Autodesk Fusion 360 part; units mm, degrees
sketch "Sketch1" plane through (0, 0, 0) normal (0, 0, 1) x (1, 0, 0) in component "Case "
  line L0 (0, 0) -> (117.5, 0)
  line L1 (117.5, 0) -> (117.5, -47.5)
  line L2 (117.5, -47.5) -> (62.4309, -113.1288)
  line L3 (0, 0) -> (0, -75)
  line L4 (0, -75) -> (62.4309, -113.1288)
  line L5 (0, -66.2119) -> (67.3065, -107.3183)
  line L6 (55.9577, -109.1753) -> (117.5, -35.8321)
  line L7 (0, -7.5) -> (117.5, -7.5)
  line L8 (110, 0) -> (110, -56.4382)
  line L9 (117.5, -47.5) -> (0, -47.5)
  dimension "d3" = 140
  dimension "d11" = 7.5
  dimension "d12" = 7.5
  dimension "d13" = 7.5
  dimension "d14" = 7.5
  dimension "d15" = 110
  dimension "d16" = 47.5
  dimension "d17" = 18.7119
  dimension "d18" = 75
extrude "Extrude1" add sketch "Sketch1" along normal blind 5
extrude "Extrude2" cut 1 faces at (39.1667, -40.8333, 5) along direction (0, 0, -1) blind 3
extrude "Extrude1'" [suppressed] in component "Case "
extrude "Extrude3" [suppressed] in component "Case "
sketch "Sketch2" plane through (0, 0, 0) normal (0, 0, 1) x (1, 0, 0) in component "Case "
  line L0 (0, 31.2783) -> (117.5, 31.2783)
  line L1 (117.5, 31.2783) -> (117.5, 78.7783)
  line L2 (117.5, 78.7783) -> (62.4311, 144.4069)
  line L3 (0, 31.2783) -> (0, 106.2783)
  line L4 (0, 106.2783) -> (62.4311, 144.4069)
  dimension "d23" = 117.5
  dimension "d24" = 47.5
  dimension "d25" = 85.672
  dimension "d29" = 75
  dimension "d31" = 140
  dimension "d32" = 73.1535
extrude "Extrude4" [suppressed] in component "Case "
extrude "Extrude5" [suppressed] in component "Case "
extrude "Extrude2'" [suppressed] in component "Case "
component "Case " placed x (1, 0, 0) y (0, 1, 0) z (0, 0, 1) at (0, 0, 0)
Can you work these out from the model? Positions are in its coordinate system, mm. Round coordinates to 2 decimals unless told otherwise and drop trailing zeros. Order: outer loops, then holes, each group sorted by start corner. A loop starts at its lowest first (then second) coordinate and runs counter-clockwise, first axis right, second up. Notation, with made-up numbers: (16.5, 81.25) -> (28.5, 81.25) arc R17 ccw to (28.5, 91.25) -> close; hole circle Ø9 at (32.25, 64.25). An arc over 180 degrees is marked (long way). Return JSON: item names as keys, results as strings. Group by question number.
1. I need wall thicknesses on line 1 (Y direction, x = 22, z = 0.1); line 2 (X direction, y = -76, z = 1.3); line 3 (Y direction, x = 52, z = 0.55). Which ranges of each line are inside material? Lowest first, please. Write a range as [from, to].
2. If we section it at A-A, the plane z = 1.4: Write out the boundary of the cut face in (x, y), then the cut area to 3 significant figures.
3. If we section it at C-C, the plane y = -50.5: Write out the boundary of the cut face in (x, z).
4. Will this pin go through, and if not, where does the flat tip stop? pin 1 (1 mm diameter, centred on y = -60.5, z = 1, fed in from +X).
5. We'd pull the mould along Z, two halves only. Please class faces 1 (the face through (58, -43, 2)), 2 (the face through (30.78, -93.8, 0.99)), 3 (the face through (58, -43, 0)): released by +Z, released by -Z, zero draft, split by the parting line, or undercut.
6. If we section it at B-B, the plane x = 100.5: Write out the boundary of the cut face in (y, z).
Output values:
{
 "1": {"line 1": "[-88.44, 0]", "line 2": "[1.64, 93.59]", "line 3": "[-106.76, 0]"},
 "2": {"outline": "(0, -75) -> (62.43, -113.13) -> (117.5, -47.5) -> (117.5, 0) -> (0, 0) -> close", "area": "10,300 mm²"},
 "3": {"outline": "(0, 0) -> (114.98, 0) -> (114.98, 2) -> (0, 2) -> close"},
 "4": {"pin 1": "x = 107.01"},
 "5": {"face 1": "released by +Z", "face 2": "zero draft", "face 3": "released by -Z"},
 "6": {"outline": "(-67.76, 0) -> (0, 0) -> (0, 2) -> (-67.76, 2) -> close"}
}
